Check sheet for the drawn part. Datum: minimum x, y, z corner. Units: mm. Give positions to 0.01 mm unless a question says otherwise; leave off trailing zeros. Order: outer loops, then holes, each group sorted by start corner. A loop starts at its lowest first (then second) coordinate and runs counter-clockwise, first axis right, second up. Notation, with made-up numbers: (-15, -25.5) -> (28, -25.5) arc R18 cw to (28, -20.5) -> close; hole circle Ø9 at (18.5, 75). An arc over 180 degrees is marked (long way). One line per question, with ' | ' between items. Start each with the question number.
Q1. Go/stop test with a flat-tipped pin: pin 1 (2.5 mm diameter, centred on x = 44.34, z = 52.76, fed in from -Y). Record where the tip stops, or that it passes through.
Q2. Section check A-A on y = 1.35. Give the number of separate pieces and of enclosed holes in the cut face, plus the area to 3 significant figures.
Q3. Section check C-C on x = 20.5. Record the cut outline in (y, z), plus the area to 3 significant figures.
Q4. Material ranges on probe 1 along Z at (x, y) = (58, 1.25); probe 2 along X at (y, z) = (1.7, 59.5); probe 3 along X at (y, z) = (2.7, 77), recorded low to high. Write a range as [from, to].
Q5. Section check B-B on z = 12. Record the cut outline in (x, y).
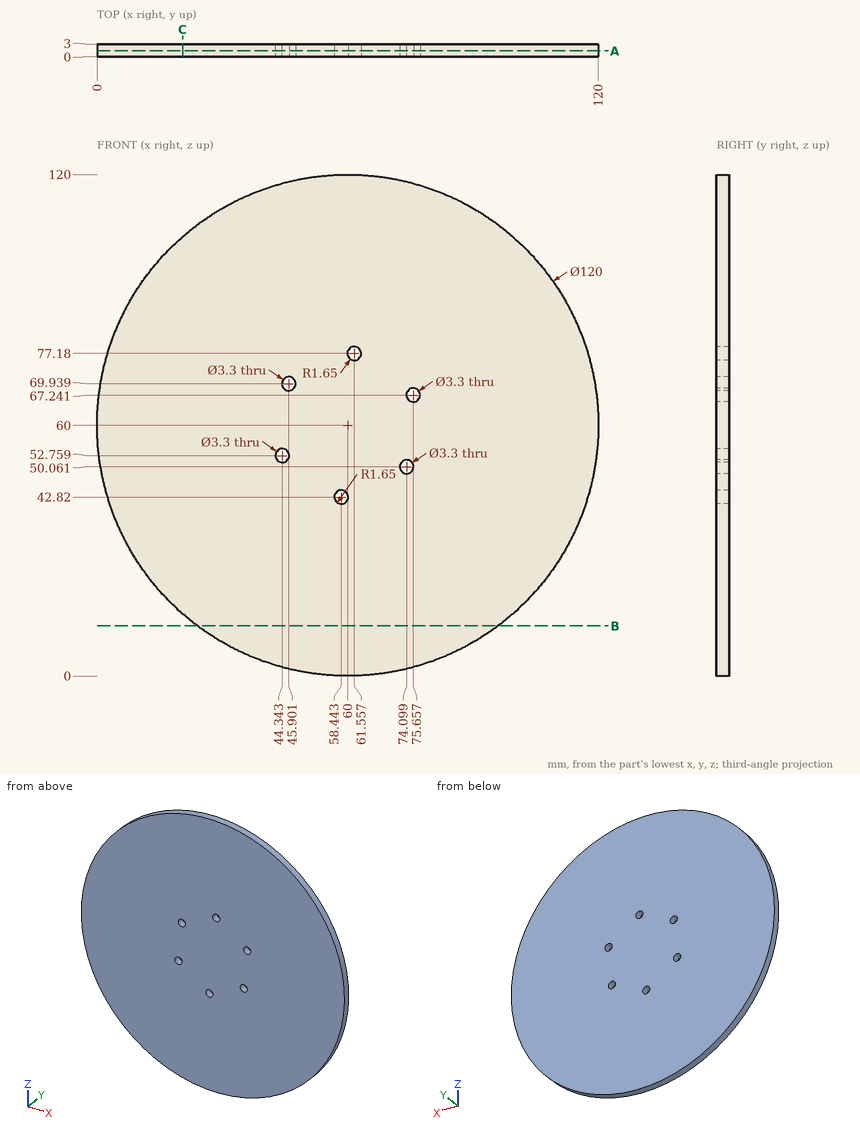
Filled in:
1) pin 1: through
2) separate pieces: 1 | enclosed holes: 6 | area: 11,300 mm²
3) outline: (0, 14.84) -> (3, 14.84) -> (3, 105.16) -> (0, 105.16) -> close | area: 271 mm²
4) probe 1: [0.03, 41.23], [44.41, 119.97] | probe 2: [0, 120] | probe 3: [2.46, 59.92], [63.2, 117.54]
5) outline: (24, 0) -> (96, 0) -> (96, 3) -> (24, 3) -> close
